Part print with two shaded views. Sizes in mm from the minimum x, y, z corner. Round coordinates to 2 decimals unless told otherwise and drop trailing zeros. Loops run counter-clockwise (first coordinate to the right, second up) from the corner with the lowest first, then second, coordinate; pieces in that order, holes last. Notation, with made-up numbers: M -1.75,86.5 L 34.25,86.5 A15 cw 34.25,112.5 Z; hole C 3.5,-17 d7. An arc over 180 degrees is marked long. Put each result on its own line as item: value. Start each with the question number.
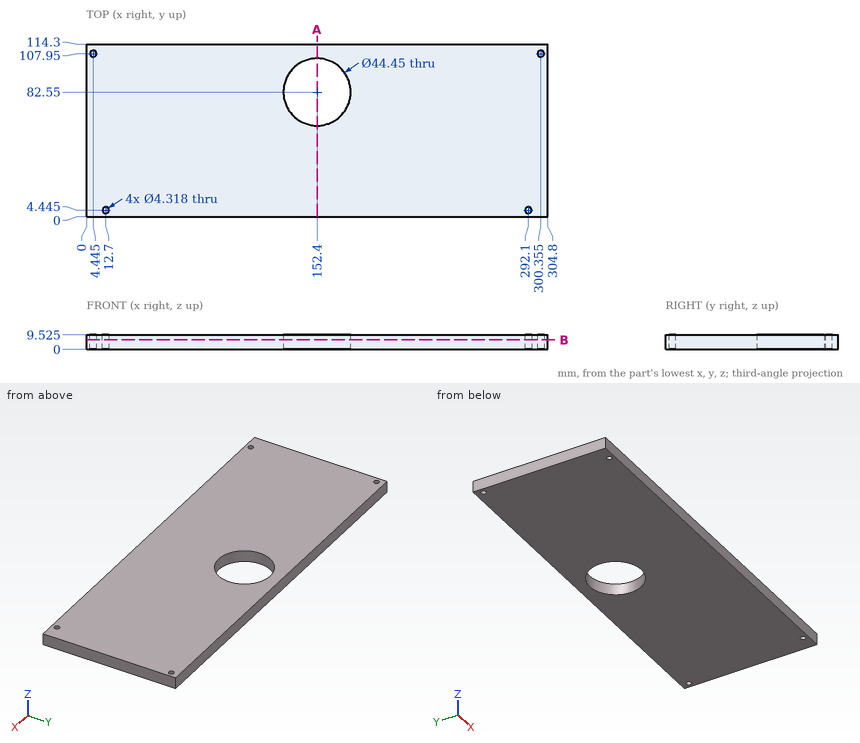
(1) Cut at B-B on z = 6.25. List the corners of the cut face in (x, y) (3 decimals).
(2) Drill centre lines: line 1 along X through (y, z) = (107.95, 6.5); line 2 along Y through (x, z) = (292.1, 7.5); line 3 along X through (y, z) = (82, 2.25). Where is each one in solid material? Low to high.
(3) Cut at A-A on x = 152.4. List the corners of the cut face in (y, z) (3 decimals).
(4) Flat gauge pin, fed straight in: pin 1 Ø4 at (x, y) = (4.445, 107.95) entering from -Z. Where does the tip first touch, or does it go through?
Taken from the geometry:
1. outline: M 0,0 L 304.8,0 L 304.8,114.3 L 0,114.3 Z; hole C 4.445,107.95 d4.318; hole C 12.7,4.445 d4.318; hole C 152.4,82.55 d44.45; hole C 292.1,4.445 d4.318; hole C 300.355,107.95 d4.318
2. line 1: 0 to 2.29, 6.6 to 298.2, 302.51 to 304.8
2. line 2: 0 to 2.29, 6.6 to 114.3
2. line 3: 0 to 130.18, 174.62 to 304.8
3. outline: M 0,0 L 60.325,0 L 60.325,9.525 L 0,9.525 Z; M 104.775,0 L 114.3,0 L 114.3,9.525 L 104.775,9.525 Z
4. pin 1: through
